Check sheet for the modelled part. Datum: model origin and axes. Units: mm. A direction names the side the tool comes from. Give positions to 0.01 mm unless a question says otherwise; leave off trailing zeros. Write each loop counter-clockwise with the first axis right and the second up, starting at its lowest first coordinate (ties: lowest second). Pieces come first, ordered by that corner, then holes. Notation, with made-up numbers: (-36, 59) -> (-24, 59) arc R7 ccw to (-24, 69) -> close; hole circle Ø1 at (81, 8). An arc over 180 degrees is marked (long way). Answer as a JSON object with one key per item and string values.
from build123d import *

# Parameters (mm, degrees)
SKETCH_W        = 25
SKETCH_H        = 25
PAD_DEPTH       = 12.5
THICKNESS_T     = -3.5
SKETCH001_W     = 18
SKETCH001_H     = 9
POCKET_DEPTH    = 3.5
PAD001_DEPTH    = 50
CHAMFER_SIZE    = 1
SKETCH003_W     = 18
SKETCH003_H     = 9
POCKET001_DEPTH = 3.5
PAD002_DEPTH    = 50
CHAMFER001_SIZE = 1
SKETCH005_W     = 18
SKETCH005_H     = 9
POCKET002_DEPTH = 3.5
PAD003_DEPTH    = 50
CHAMFER002_SIZE = 1
FILLET_R        = 2
FILLET001_R     = 2
FILLET002_R     = 2
FILLET003_R     = 2
FILLET004_R     = 2


with BuildPart() as part:
    # Sketch → Pad (new body)
    with BuildSketch(Plane.XY):
        Rectangle(SKETCH_W, SKETCH_H)
    extrude(amount=PAD_DEPTH)

    # Thickness
    thickness_openings = [part.faces().sort_by_distance(p)[0] for p in [
        (0, 0, 12.5),
    ]]
    offset(amount=THICKNESS_T, openings=thickness_openings, kind=Kind.INTERSECTION)

    # Sketch001 (on Face2 of Thickness) → Pocket (cut)
    with BuildSketch(Plane.XZ.offset(12.5)):
        with Locations((0, 8)):
            Rectangle(SKETCH001_W, SKETCH001_H)
    extrude(amount=-POCKET_DEPTH, mode=Mode.SUBTRACT)

    # Sketch002 (on Face3 of Pocket) → Pad001 (join)
    with BuildSketch(Plane.XZ.offset(12.5)):
        Polygon((-10.25, 12.5), (-10.25, 2.25), (10.25, 2.25), (10.25, 12.5), (9, 12.5), (9, 3.5), (-9, 3.5), (-9, 12.5), align=None)
    extrude(amount=PAD001_DEPTH)

    # Chamfer
    chamfer_edges = [part.edges().sort_by_distance(p)[0] for p in [
        (0, -62.5, 2.25),
        (10.25, -37.5, 2.25),
        (-10.25, -37.5, 2.25),
        (10.25, -62.5, 7.375),
        (-10.25, -62.5, 7.375),
    ]]
    chamfer(chamfer_edges, length=CHAMFER_SIZE)

    # Sketch003 (on Face6 of Chamfer) → Pocket001 (cut)
    with BuildSketch(Plane.YZ.offset(12.5)):
        with Locations((0, 8)):
            Rectangle(SKETCH003_W, SKETCH003_H)
    extrude(amount=-POCKET001_DEPTH, mode=Mode.SUBTRACT)

    # Sketch004 (on Face6 of Pocket001) → Pad002 (join)
    with BuildSketch(Plane.YZ.offset(12.5)):
        Polygon((10.25, 12.5), (10.25, 2.25), (-10.25, 2.25), (-10.25, 12.5), (-9, 12.5), (-9, 3.5), (9, 3.5), (9, 12.5), align=None)
    extrude(amount=PAD002_DEPTH)

    # Chamfer001
    chamfer001_edges = [part.edges().sort_by_distance(p)[0] for p in [
        (37.5, -10.25, 2.25),
        (62.5, -10.25, 7.375),
        (62.5, 0, 2.25),
        (62.5, 10.25, 7.375),
        (37.5, 10.25, 2.25),
    ]]
    chamfer(chamfer001_edges, length=CHAMFER001_SIZE)

    # Sketch005 → Pocket002 (cut)
    with BuildSketch(Plane(origin=(0, 12.5, 0), x_dir=(-1, 0, 0), z_dir=(0, 1, 0))):
        with Locations((0, 8)):
            Rectangle(SKETCH005_W, SKETCH005_H)
    extrude(amount=-POCKET002_DEPTH, mode=Mode.SUBTRACT)

    # Sketch006 (on Face6 of Pocket002) → Pad003 (join)
    with BuildSketch(Plane(origin=(0, 12.5, 0), x_dir=(-1, 0, 0), z_dir=(0, 1, 0))):
        Polygon((10.25, 12.5), (10.25, 2.25), (-10.25, 2.25), (-10.25, 12.5), (-9, 12.5), (-9, 3.5), (9, 3.5), (9, 12.5), align=None)
    extrude(amount=PAD003_DEPTH)

    # Chamfer002
    chamfer002_edges = [part.edges().sort_by_distance(p)[0] for p in [
        (-10.25, 37.5, 2.25),
        (0, 62.5, 2.25),
        (-10.25, 62.5, 7.375),
        (10.25, 62.5, 7.375),
        (10.25, 37.5, 2.25),
    ]]
    chamfer(chamfer002_edges, length=CHAMFER002_SIZE)

    # Fillet
    fillet_edges = [part.edges().sort_by_distance(p)[0] for p in [
        (-9, 37.5, 3.5),
    ]]
    fillet(fillet_edges, radius=FILLET_R)

    # Fillet001
    fillet001_edges = [part.edges().sort_by_distance(p)[0] for p in [
        (9, 37.5, 3.5),
    ]]
    fillet(fillet001_edges, radius=FILLET001_R)

    # Fillet002
    fillet002_edges = [part.edges().sort_by_distance(p)[0] for p in [
        (37.5, 9, 3.5),
    ]]
    fillet(fillet002_edges, radius=FILLET002_R)

    # Fillet003
    fillet003_edges = [part.edges().sort_by_distance(p)[0] for p in [
        (9, -37.5, 3.5),
    ]]
    fillet(fillet003_edges, radius=FILLET003_R)

    # Fillet004
    fillet004_edges = [part.edges().sort_by_distance(p)[0] for p in [
        (37.5, -9, 3.5),
    ]]
    fillet(fillet004_edges, radius=FILLET004_R)


solid = part.part
1. Scan line: L1, parallel to X at y = -19, z = 11. Record every from-to range of solid material in increasing order. Write a range as [from, to].
Determined:
{"L1": "[-10.25, -9], [9, 10.25]"}
2. Go/stop test with flat-tipped pins: P1, Ø7.5, axis at y = 43, z = 7.5, coming from the -X side; P2, Ø1.5, axis at x = 13, z = 1.5, coming from the -Y side; P3, Ø1.5, axis at x = -2, z = 2, coming from the -Y side. Record where each tip stops, or that it passes through.
Determined:
{"P1": "x = -10.25", "P2": "y = -12.5", "P3": "y = -62"}
3. Sectioned sample at A-A, the plane z = 8. State how many separate pieces and enclosed holes the cut face has, plus the area to 3 significant figures.
Determined:
{"separate pieces": "3", "enclosed holes": "0", "area": "484 mm^2"}
4. Sectioned sample at D-D, the plane x = 3. Enter the section's corners in (y, z).
Determined:
{"outline": "(-62.5, 3.25) -> (-61.5, 2.25) -> (-12.5, 2.25) -> (-12.5, 0) -> (12.5, 0) -> (12.5, 2.25) -> (61.5, 2.25) -> (62.5, 3.25) -> (62.5, 3.5) -> (-62.5, 3.5) -> close"}
5. Sectioned sample at C-C, the plane y = 4.5. Enter the section's corners in (x, z), plus the area to 3 significant figures.
Determined:
{"outline": "(-12.5, 0) -> (12.5, 0) -> (12.5, 2.25) -> (61.5, 2.25) -> (62.5, 3.25) -> (62.5, 3.5) -> (-7, 3.5) arc R2 cw to (-9, 5.5) -> (-9, 12.5) -> (-12.5, 12.5) -> close", "area": "182 mm^2"}
6. Mould release check, pull along X, two halves, no side actions. Record for faces 6 (the face through (37, -10.25, 8)), 7 (the face through (12.5, 0, 2)), 8 (the face through (12, 0, 3.5)), 9 (the face through (-12.5, 0, 6)): released by +X, released by -X, zero draft, split by the parting line, or undercut.
Determined:
{"face 6": "zero draft", "face 7": "released by +X", "face 8": "undercut", "face 9": "released by -X"}
7. Access from +Z, -Z, +X, -X, +Y, -Y to the whole of each face (thin tool, end or side, straight path). Record for faces 1 (the face through (10.25, 37, 8)), 2 (the face through (35, 9, 9)), 3 (the face through (9, 35, 9)), 4 (the face through (0, 37, 2.25)), 5 (the face through (0, -37, 2.25)).
Determined:
{"face 1": "+Z, -Z, +X, +Y", "face 2": "+Z, +X", "face 3": "+Z, +Y, -Y", "face 4": "-Z, +X, -X, +Y", "face 5": "-Z, +X, -X, -Y"}
8. Sectioned sample at B-B, the plane x = 46.5. Enter the section's corners in (y, z), plus the area to 3 significant figures.
Determined:
{"outline": "(-10.25, 3.25) -> (-9.25, 2.25) -> (9.25, 2.25) -> (10.25, 3.25) -> (10.25, 12.5) -> (9, 12.5) -> (9, 5.5) arc R2 cw to (7, 3.5) -> (-7, 3.5) arc R2 cw to (-9, 5.5) -> (-9, 12.5) -> (-10.25, 12.5) -> close", "area": "48.8 mm^2"}
